from build123d import *

# Parameters (mm, degrees)
AUFSATZ_LINEAR_AUSTRAGEN1_DEPTH                      = 15
AUFSATZ_LINEAR_AUSTRAGEN2_DEPTH                      = 2
FORMSENKUNG_F_R_M3_SENKSCHRAUBE_MIT_INNE_D           = 3.4
FORMSENKUNG_F_R_M3_SENKSCHRAUBE_MIT_INNE_DEPTH       = 10
FORMSENKUNG_F_R_M3_SENKSCHRAUBE_MIT_INNE_CSINK_D     = 6.94
FORMSENKUNG_F_R_M3_SENKSCHRAUBE_MIT_INNE_CSINK_ANGLE = 90
FORMSENKUNG_F_R_M3_SENKSCHRAUBE_MIT_INNE_TIP         = 1.021463052


with BuildPart() as part:
    # Skizze1 → Aufsatz-Linear austragen1 (new body)
    with BuildSketch(Plane(origin=(0, 0, 0), x_dir=(1, 0, 0), z_dir=(0, 1, 0))):
        Polygon((0, 0), (22, 0), (22, -30), (104.5, -30), (104.5, 0), (126.5, 0), (126.5, -2), (106.5, -2), (106.5, -32), (20, -32), (20, -2), (0, -2), align=None)
    extrude(amount=AUFSATZ_LINEAR_AUSTRAGEN1_DEPTH)

    # Skizze2 → Aufsatz-Linear austragen2 (add)
    with BuildSketch(Plane.XZ):
        Polygon((22, 0), (32, 0), (32, 25), (94.5, 25), (94.5, 0), (104.5, 0), (104.5, 30), (22, 30), align=None)
    extrude(amount=-AUFSATZ_LINEAR_AUSTRAGEN2_DEPTH)

    # Formsenkung für M3 Senkschraube mit Innensechskant1
    with Locations(Plane.XY.offset(2)):
        with Locations((10, 7.5), (116.5, 7.5)):
            CounterSinkHole(FORMSENKUNG_F_R_M3_SENKSCHRAUBE_MIT_INNE_D / 2, FORMSENKUNG_F_R_M3_SENKSCHRAUBE_MIT_INNE_CSINK_D / 2, depth=FORMSENKUNG_F_R_M3_SENKSCHRAUBE_MIT_INNE_DEPTH, counter_sink_angle=FORMSENKUNG_F_R_M3_SENKSCHRAUBE_MIT_INNE_CSINK_ANGLE)
            with Locations((0, 0, -(FORMSENKUNG_F_R_M3_SENKSCHRAUBE_MIT_INNE_DEPTH + FORMSENKUNG_F_R_M3_SENKSCHRAUBE_MIT_INNE_TIP / 2))):  # 118° drill point
                Cone(0, FORMSENKUNG_F_R_M3_SENKSCHRAUBE_MIT_INNE_D / 2, FORMSENKUNG_F_R_M3_SENKSCHRAUBE_MIT_INNE_TIP, mode=Mode.SUBTRACT)


solid = part.part
Check sheet for the modelled part. Datum: model origin and axes. Units: mm. A direction names the side the tool comes from. Coordinates: 2 decimals unless noted, no trailing zeros. Write each loop counter-clockwise with the first axis right and the second up, starting at its lowest first coordinate (ties: lowest second). Pieces come first, ordered by that corner, then holes.
Item 1: Cross-section at C-C on y = 7.5. Record the boundary of the cut face in (x, z), then the cut area to 3 significant figures.
Numbers:
outline: (0, 0) - (8.3, 0) - (8.3, 0.23) - (6.53, 2) - (0, 2) - close; (11.7, 0) - (22, 0) - (22, 30) - (104.5, 30) - (104.5, 0) - (114.8, 0) - (114.8, 0.23) - (113.03, 2) - (106.5, 2) - (106.5, 32) - (20, 32) - (20, 2) - (13.47, 2) - (11.7, 0.23) - close; (118.2, 0) - (126.5, 0) - (126.5, 2) - (119.97, 2) - (118.2, 0.23) - close
area: 353 mm2
Item 2: Cross-section at B-B on z = 5. Record the boundary of the cut face in (x, y), then the cut area to 3 significant figures.
Numbers:
outline: (20, 0) - (32, 0) - (32, 2) - (22, 2) - (22, 15) - (20, 15) - close; (94.5, 0) - (106.5, 0) - (106.5, 15) - (104.5, 15) - (104.5, 2) - (94.5, 2) - close
area: 100 mm2
Item 3: Cross-section at D-D on z = 28.5. Record the boundary of the cut face in (x, y), then the cut area to 3 significant figures.
Numbers:
outline: (20, 0) - (106.5, 0) - (106.5, 15) - (104.5, 15) - (104.5, 2) - (22, 2) - (22, 15) - (20, 15) - close
area: 225 mm2
Item 4: Access from +Z, -Z, +X, -X, +Y, -Y to the whole of each face (thin tool, end or side, straight path). Record for faces 1 (the face through (63, 1, 25)), 2 (the face through (104.5, 8, 15)), 3 (the face through (106.5, 7, 17)).
Numbers:
face 1: -Z, +Y, -Y
face 2: -Z, +Y
face 3: +Z, +X, +Y, -Y
Item 5: Scan lines: probe 1 along X at (y, z) = (7.5, 0.15); probe 2 along X at (y, z) = (2.75, 11.5); probe 3 along X at (y, z) = (1.25, 15). Record each from-to range of solid material in increasing order.
Numbers:
probe 1: x = 0 to 8.3, 11.7 to 22, 104.5 to 114.8, 118.2 to 126.5
probe 2: x = 20 to 22, 104.5 to 106.5
probe 3: x = 20 to 32, 94.5 to 106.5
Item 6: Depth check by flat-ended pin: pin 1 Ø4 at (y, z) = (8.5, 3.5) entering from -X; pin 2 Ø4.5 at (x, y) = (5, 10) entering from +Z; pin 3 Ø1.5 at (x, y) = (79.5, 7.5) entering from -Z; pin 4 Ø7.5 at (y, z) = (10.5, 23) entering from +X. Enter the tip coordinate at first touch or a pass-through.
Numbers:
pin 1: stops at x = 0
pin 2: stops at z = 2
pin 3: stops at z = 30
pin 4: stops at x = 106.5
Item 7: Cross-section at A-A on x = 116.5. Record the boundary of the cut face in (y, z), then the cut area to 3 significant figures.
Numbers:
outline: (0, 0) - (5.8, 0) - (5.8, 0.23) - (4.03, 2) - (0, 2) - close; (9.2, 0) - (15, 0) - (15, 2) - (10.97, 2) - (9.2, 0.23) - close
area: 20.1 mm2
